```python
from build123d import *

# Parameters (mm, degrees)
SKETCH1_W           = 420
SKETCH1_H           = 150
BOSS_EXTRUDE1_DEPTH = 20
SKETCH2_W           = 10
SKETCH2_H           = 150
BOSS_EXTRUDE3_DEPTH = 20
FILLET1_R           = 10
FILLET2_R           = 10
FILLET3_R           = 10
FILLET4_R           = 10
SKETCH3_R           = 65
SKETCH3_R_2         = 50
BOSS_EXTRUDE4_DEPTH = 200
FILLET5_R           = 10
CUT_EXTRUDE1_START  = -327
SKETCH4_R           = 50
CUT_EXTRUDE1_DEPTH  = 327


with BuildPart() as part:
    # Sketch1 → Boss-Extrude1 (new body)
    with BuildSketch(Plane(origin=(0, 0, 0), x_dir=(1, 0, 0), z_dir=(0, 1, 0))):
        Rectangle(SKETCH1_W, SKETCH1_H)
    extrude(amount=BOSS_EXTRUDE1_DEPTH)

    # Sketch2 → Boss-Extrude3 (add)
    with BuildSketch(Plane.XZ):
        with Locations((-205, 0)):
            Rectangle(SKETCH2_W, SKETCH2_H)
        with Locations((-175, 0)):
            Rectangle(SKETCH2_W, SKETCH2_H)
        with Locations((205, 0)):
            Rectangle(SKETCH2_W, SKETCH2_H)
        with Locations((175, 0)):
            Rectangle(SKETCH2_W, SKETCH2_H)
    extrude(amount=BOSS_EXTRUDE3_DEPTH)

    # Fillet1
    fillet1_edges = [part.edges().sort_by_distance(p)[0] for p in [
        (-170, 0, 0),
    ]]
    fillet(fillet1_edges, radius=FILLET1_R)

    # Fillet2
    fillet2_edges = [part.edges().sort_by_distance(p)[0] for p in [
        (170, 0, 0),
    ]]
    fillet(fillet2_edges, radius=FILLET2_R)

    # Fillet3
    fillet3_edges = [part.edges().sort_by_distance(p)[0] for p in [
        (210, 20, 0),
    ]]
    fillet(fillet3_edges, radius=FILLET3_R)

    # Fillet4
    fillet4_edges = [part.edges().sort_by_distance(p)[0] for p in [
        (-210, 20, 0),
    ]]
    fillet(fillet4_edges, radius=FILLET4_R)

    # Sketch3 → Boss-Extrude4 (add)
    with BuildSketch(Plane(origin=(0, 20, 0), x_dir=(1, 0, 0), z_dir=(0, 1, 0))):
        with Locations(Location((0, 0, 0), (0, 0, 90))):
            Circle(SKETCH3_R)
        with Locations(Location((0, 0, 0), (0, 0, 270))):
            Circle(SKETCH3_R_2, mode=Mode.SUBTRACT)
    extrude(amount=BOSS_EXTRUDE4_DEPTH)

    # Fillet5
    fillet5_edges = [part.edges().sort_by_distance(p)[0] for p in [
        (0, 20, 65),
    ]]
    fillet(fillet5_edges, radius=FILLET5_R - 0.0001)  # a hair under: the kernel refuses the full size

    # Sketch4 → Cut-Extrude1 (cut)
    with BuildSketch(Plane(origin=(0, 220, 0), x_dir=(1, 0, 0), z_dir=(0, 1, 0)).offset(CUT_EXTRUDE1_START)):
        with Locations(Location((0, 0, 0), (0, 0, 90))):
            Circle(SKETCH4_R)
    extrude(amount=CUT_EXTRUDE1_DEPTH, mode=Mode.SUBTRACT)


solid = part.part
```
The model under review builds one solid part; all positions refer to its coordinate system, in mm. A direction names the side the tool comes from. Coordinates: 2 decimals unless noted, no trailing zeros. Write each loop counter-clockwise with the first axis right and the second up, starting at its lowest first coordinate (ties: lowest second). Pieces come first, ordered by that corner, then holes.
1) We need section C-C on y = 93.5. State the section outline as (x, z) points, then the cut area to 3 significant figures.
2) Clearance check with flat-ended pins moving along their axes: pin 1 Ø12 at (x, y) = (55.5, 72.5) entering from -Z; pin 2 Ø6 at (x, z) = (21.5, 55) entering from -Y; pin 3 Ø6 at (x, z) = (50, -56) entering from +Y. State where each tip first meets the part, or that it passes through.
3) To check wall thickness, follow probe 1 along X at (y, z) = (158, 0); probe 2 along Y at (x, z) = (-131.5, -48); probe 3 along Y at (x, z) = (50, 39). State the ranges of each line that lie inside material, in increasing order.
4) The part is to be moulded in two halves that separate along X. For faces 3 (the face through (-47, 20, 66)), 4 (the face through (-166.99, -2.85, 1.05)), 5 (the face through (210, -5, 1)), say which applies: pulls with the +X half, pulls with the -X half, needs draft (parallel to the pull), parting line crosses it, or undercut.
5) Machinability: for faces 1 (the face through (-206.99, 17.15, -1.05)), 2 (the face through (-200, -10, -1)), which of the approach directions +Z, -Z, +X, -X, +Y, -Y give a long, thin tool a straight path to every point of the face, cutting with its end or side? Answer none if there is none.
Answer list:
1. outline: circle Ø130 at (0, 0); hole circle Ø100 at (0, 0)
1. area: 5,420 mm2
2. pin 1: stops at z = -42.13
2. pin 2: stops at y = 0
2. pin 3: stops at y = 20.44
3. probe 1: x = -65 to -50, 50 to 65
3. probe 2: y = 0 to 20
3. probe 3: y = 0 to 220
4. face 3: needs draft
4. face 4: undercut
4. face 5: pulls with the +X half
5. face 1: +Z, -Z, -X, +Y
5. face 2: +Z, -Z, -Y
